Design review of the part shown in the three views and the two pictorial views. Dimensions are in mm from the part's minimum x, y and z. Give positions to 0.01 mm unless a question says otherwise; leave off trailing zeros. Order: outer loops, then holes, each group sorted by start corner. A loop starts at its lowest first (then second) coordinate and runs counter-clockwise, first axis right, second up. Notation, with made-up numbers: (4.5, 86) -> (10.5, 86) arc R23 ccw to (10.5, 96) -> close; hole circle Ø6 at (7, 43). An arc over 180 degrees is marked (long way). Use one line per item in the form item = value.
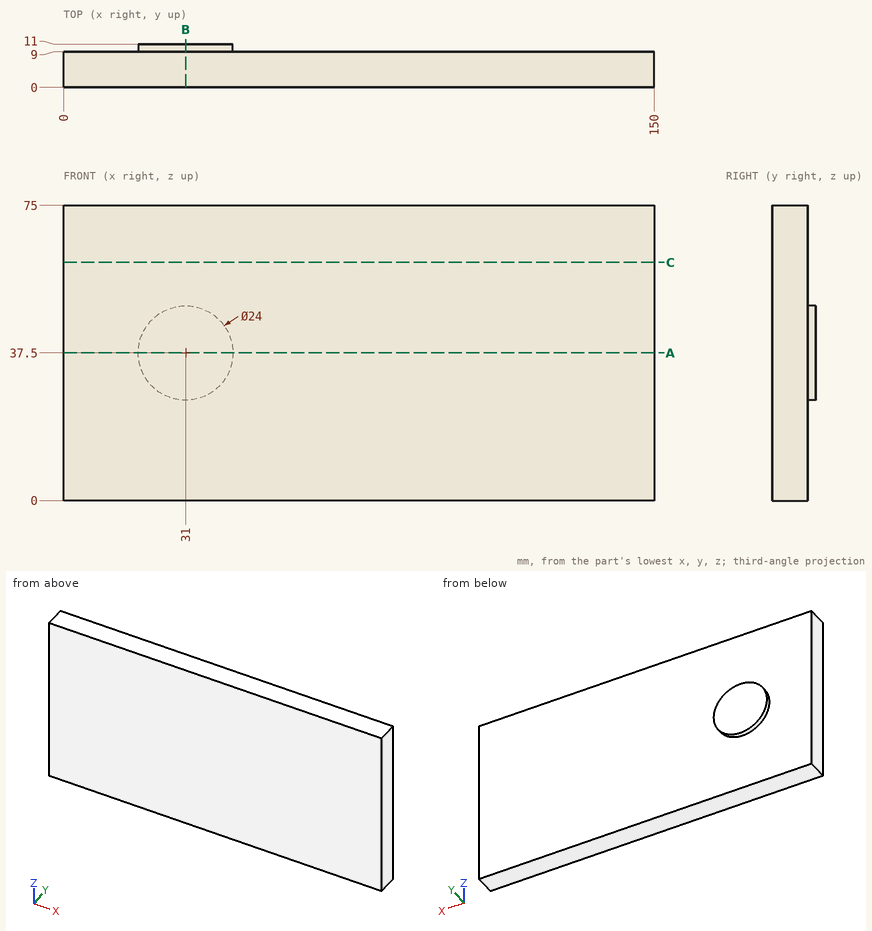
1. For pin 1 Ø8 at (x, z) = (36.5, 21.5) entering from +Y; pin 2 Ø1 at (y, z) = (10, 62.5) entering from -X, all flat-tipped, find the tip position at first contact; note any pin that passes through.
Values:
pin_1 = 9
pin_2 = through
2. Add section C-C on z = 60.5. Give the boundary of the cut face in (x, y).
Values:
outline = (0, 0) -> (150, 0) -> (150, 9) -> (0, 9) -> close
3. For L1, parallel to Y at x = 52.5, z = 66.5; L2, parallel to X at y = 10.25, z = 48, list the stretches that pass through material, from the lowest coordinate up.
Values:
L1 = 0 to 9
L2 = 25.19 to 36.81
4. Add section B-B on x = 31. Give the boundary of the cut face in (y, z).
Values:
outline = (0, 0) -> (9, 0) -> (9, 25.5) -> (11, 25.5) -> (11, 49.5) -> (9, 49.5) -> (9, 75) -> (0, 75) -> close
5. Add section A-A on z = 37.5. Give the boundary of the cut face in (x, y), then the cut area to 3 significant figures.
Values:
outline = (0, 0) -> (150, 0) -> (150, 9) -> (43, 9) -> (43, 11) -> (19, 11) -> (19, 9) -> (0, 9) -> close
area = 1,400 mm^2
